from build123d import *

# Parameters (mm, degrees)
SKETCH1_W           = 35
SKETCH1_H           = 2
BOSS_EXTRUDE1_DEPTH = 14
SKETCH2_R           = 1.75
CUT_EXTRUDE1_DEPTH  = 14


with BuildPart() as part:
    # Sketch1 → Boss-Extrude1 (new body)
    with BuildSketch(Plane(origin=(0, 0, 0), x_dir=(1, 0, 0), z_dir=(0, 1, 0))):
        Rectangle(SKETCH1_W, SKETCH1_H)
    extrude(amount=BOSS_EXTRUDE1_DEPTH)

    # Sketch2 → Cut-Extrude1 (cut)
    with BuildSketch(Plane.XY.offset(1)):
        with Locations((-14, 5)):
            Circle(SKETCH2_R)
        with Locations((14, 5)):
            Circle(SKETCH2_R)
    extrude(amount=-CUT_EXTRUDE1_DEPTH, mode=Mode.SUBTRACT)


solid = part.part
Verification items for the finished model (mm, model axes). Coordinates: 2 decimals unless noted, no trailing zeros. Loops run counter-clockwise (first coordinate to the right, second up) from the corner with the lowest first, then second, coordinate; pieces in that order, holes last. Notation, with made-up numbers: (26, -27.75) -> (56, -27.75) arc R12 cw to (56, -23.75) -> close; hole circle Ø6 at (76, 68.25). An arc over 180 degrees is marked (long way). Write each question's results on one line, items separated by ' | '.
Item 1: Section check A-A, the plane x = -14. Enter the section's corners in (y, z).
Found:
outline: (0, -1) -> (3.25, -1) -> (3.25, 1) -> (0, 1) -> close; (6.75, -1) -> (14, -1) -> (14, 1) -> (6.75, 1) -> close
Item 2: Section check B-B, the plane z = 0. Enter the section's corners in (x, y).
Found:
outline: (-17.5, 0) -> (17.5, 0) -> (17.5, 14) -> (-17.5, 14) -> close; hole circle Ø3.5 at (-14, 5); hole circle Ø3.5 at (14, 5)
Item 3: Material ranges on L1, parallel to Y at x = -14, z = -0.25; L2, parallel to X at y = 6.25, z = -0.4; L3, parallel to X at y = 5.5, z = -0.6, recorded low to high.
Found:
L1: y = 0 to 3.25, 6.75 to 14 | L2: x = -17.5 to -15.22, -12.78 to 12.78, 15.22 to 17.5 | L3: x = -17.5 to -15.68, -12.32 to 12.32, 15.68 to 17.5
Item 4: Section check C-C, the plane y = 3.75. Enter the section's corners in (x, z), plus the area to 3 significant figures.
Found:
outline: (-17.5, -1) -> (-15.22, -1) -> (-15.22, 1) -> (-17.5, 1) -> close; (-12.78, -1) -> (12.78, -1) -> (12.78, 1) -> (-12.78, 1) -> close; (15.22, -1) -> (17.5, -1) -> (17.5, 1) -> (15.22, 1) -> close | area: 60.2 mm2
Item 5: Section check D-D, the plane y = 5.75. Enter the section's corners in (x, z).
Found:
outline: (-17.5, -1) -> (-15.58, -1) -> (-15.58, 1) -> (-17.5, 1) -> close; (-12.42, -1) -> (12.42, -1) -> (12.42, 1) -> (-12.42, 1) -> close; (15.58, -1) -> (17.5, -1) -> (17.5, 1) -> (15.58, 1) -> close
Item 6: Mould release check, pull along Y, two halves, no side actions. Record for faces 1 (the face through (0, 14, 0)), 2 (the face through (0, 7, 1)), 3 (the face through (14.81, 3.45, 0.01)): +Y half, -Y half, draft (parallel to the pull), parting line (faces both ways), or undercut.
Found:
face 1: +Y half | face 2: draft | face 3: undercut
